Part model, mm, in its own coordinate system. A direction names the side the tool comes from. Give positions to 0.01 mm unless a question says otherwise; leave off trailing zeros.
1. Probe line 1 (X direction, y = 6.5, z = 0.9); line 2 (Y direction, x = 6, z = 1.5); line 3 (Y direction, x = -5, z = 1.85). List the from-to ranges inside material, lowest first.
2. Drop flat-ended pins along their axis: pin 1 Ø2 at (x, z) = (-1.5, 0) entering from -Y; pin 2 Ø3 at (x, y) = (-6, 4.5) entering from +Z; pin 3 Ø1.5 at (x, z) = (-12, -1.5) entering from +Y. Give the stop position or say it passes through.
3. Which spindle directions (+Z, -Z, +X, -X, +Y, -Y) get a long thin tool onto all of the face, cutting with end or side? Do faces 4 (the flat face through (0, 0, -2.5)), 5 (the cylindrical face through (9.1, 6.98, 0.87)). Say none if no direction does.
4. Slice it at C-C on z = 1.1. Give the number of separate pieces and of enclosed holes in the cut face, and give its area (3 significant figures).
5. Mould opens along X. For faces 1 (the cylindrical face through (-0.18, -16.5, -1.07)), 2 (the cylindrical face through (-16.5, 0.18, -1.07)), 3 (the cylindrical face through (-2.998, -7.245, 0.873)) say: +X half, -X half, draft (parallel to the pull), parting line (faces both ways), or undercut.
from build123d import *

# Parameters (mm, degrees)
F0_W     = 36
F0_H     = 36
F1_DEPTH = 2.5
F2_R     = 3.25
F3_DEPTH = 3.3
F4_R     = 5
F5_R     = 4.99999


# Not quite as in the source:
# - a fillet or chamfer is up to 0.001 mm smaller than in the source, because OpenCascade refuses the exact size


with BuildPart() as f1:
    # F0 (on Top) → F1 (new body, symmetric)
    with BuildSketch(Plane.XY):
        Rectangle(F0_W, F0_H)
    extrude(amount=F1_DEPTH, both=True)

    # F2 (on face) → F3 (cut)
    with BuildSketch(Plane.XY.offset(2.5)):
        with Locations((-6, 6)):
            Circle(F2_R)
        with Locations((6, 6)):
            Circle(F2_R)
        with Locations((6, -6)):
            Circle(F2_R)
        with Locations((-6, -6)):
            Circle(F2_R)
    extrude(amount=-F3_DEPTH, mode=Mode.SUBTRACT)

    # F4
    f4_edges = [f1.edges().sort_by_distance(p)[0] for p in [
        (-18, -18, 0),
        (-18, 18, 0),
        (18, -18, 0),
        (18, 18, 0),
    ]]
    fillet(f4_edges, radius=F4_R)

    # F5 (radius 5 in the source; OpenCascade refuses exactly that, so slightly less here)
    f5_edges = [f1.edges().sort_by_distance(p)[0] for p in [
        (0, 18, -2.5),
    ]]
    fillet(f5_edges, radius=F5_R)


solid = f1.part
Data:
1. line 1: x = -17.74 to -9.21, -2.79 to 2.79, 9.21 to 17.74
1. line 2: y = -17.9 to -9.25, -2.75 to 2.75, 9.25 to 17.9
1. line 3: y = -17.96 to -9.09, -2.91 to 2.91, 9.09 to 17.96
2. pin 1: stops at y = -17.77
2. pin 2: stops at z = -0.8
2. pin 3: stops at y = 16.8
3. face 4: -Z, +X, -X, +Y, -Y
3. face 5: +Z
4. separate pieces: 1
4. enclosed holes: 4
4. area: 1,110 mm2
5. face 1: draft
5. face 2: -X half
5. face 3: undercut
